from build123d import *

# Parameters (mm, degrees)
SKETCH1_R           = 42
SKETCH1_R_2         = 12
BOSS_EXTRUDE1_DEPTH = 10
CHAMFER1_SIZE       = 1.5


with BuildPart() as part:
    # Sketch1 → Boss-Extrude1 (new, symmetric)
    with BuildSketch(Plane(origin=(0, 0, 0), x_dir=(1, 0, 0), z_dir=(0, 1, 0))):
        with Locations(Location((0, 0, 0), (0, 0, 270))):
            Circle(SKETCH1_R)
        with Locations(Location((0, 0, 0), (0, 0, 270))):
            Circle(SKETCH1_R_2, mode=Mode.SUBTRACT)
    extrude(amount=BOSS_EXTRUDE1_DEPTH, both=True)

    # Sketch6 → Cut-Revolve11 (revolve, cut)
    with BuildSketch(Plane.XY, mode=Mode.PRIVATE) as cut_revolve11_sk:
        with BuildLine():
            Line((-42, 5.764577254), (-42, -5.764577254))
            ThreePointArc((-42, -5.764577254), (-36.235422746, 0), (-42, 5.764577254))
        make_face()
    revolve(cut_revolve11_sk.sketch.rotate(Axis((0, 0, 0), (0, 1, 0)), 180), axis=Axis((0, 0, 0), (0, 1, 0)), mode=Mode.SUBTRACT)

    # Chamfer1
    # the kernel refuses this chamfer: 1.5 mm, written as the material it takes off along each edge
    with BuildSketch(Plane(origin=(0, -5.764577254, 0), x_dir=(0, 0, 1), z_dir=(-1, 0, 0))) as chamfer1_piece_1:
        with BuildLine():
            Line((42, -CHAMFER1_SIZE), (40.217482923, 0.282517077))
            ThreePointArc((40.217482923, 0.282517077), (41.073277318, 0.074978324), (42, 0))
            Line((42, 0), (42, -CHAMFER1_SIZE))
        make_face()
    revolve(axis=Axis((0, -5.764577254, 0), (0, 1, 0)), revolution_arc=90, mode=Mode.SUBTRACT)
    with BuildSketch(Plane(origin=(0, 5.764577254, 0), x_dir=(1, 0, 0), z_dir=(0, 0, 1))) as chamfer1_piece_2:
        with BuildLine():
            Line((40.217482923, -0.282517077), (42, CHAMFER1_SIZE))
            Line((42, CHAMFER1_SIZE), (42, 0))
            ThreePointArc((42, 0), (41.073277318, -0.074978324), (40.217482923, -0.282517077))
        make_face()
    revolve(axis=Axis((0, 5.764577254, 0), (0, 1, 0)), revolution_arc=270, mode=Mode.SUBTRACT)
    with BuildSketch(Plane(origin=(0, -10, 0), x_dir=(0, 0, 1), z_dir=(-1, 0, 0))) as chamfer1_piece_3:
        Polygon((42, CHAMFER1_SIZE), (42 - CHAMFER1_SIZE, 0), (42, 0), align=None)
    revolve(axis=Axis((0, -10, 0), (0, 1, 0)), mode=Mode.SUBTRACT)
    with BuildSketch(Plane(origin=(0, 10, 0), x_dir=(0, 0, 1), z_dir=(-1, 0, 0))) as chamfer1_piece_4:
        Polygon((42, -CHAMFER1_SIZE), (42 - CHAMFER1_SIZE, 0), (42, 0), align=None)
    revolve(axis=Axis((0, 10, 0), (0, 1, 0)), mode=Mode.SUBTRACT)
    with BuildSketch(Plane(origin=(0, -10, 0), x_dir=(0, 0, 1), z_dir=(-1, 0, 0))) as chamfer1_piece_5:
        Polygon((12 + CHAMFER1_SIZE, 0), (12, CHAMFER1_SIZE), (12, 0), align=None)
    revolve(axis=Axis((0, -10, 0), (0, 1, 0)), mode=Mode.SUBTRACT)
    with BuildSketch(Plane(origin=(0, 10, 0), x_dir=(0, 0, 1), z_dir=(-1, 0, 0))) as chamfer1_piece_6:
        Polygon((12, -CHAMFER1_SIZE), (12 + CHAMFER1_SIZE, 0), (12, 0), align=None)
    revolve(axis=Axis((0, 10, 0), (0, 1, 0)), mode=Mode.SUBTRACT)
    with BuildSketch(Plane(origin=(0, 5.764577254, 0), x_dir=(0, 0, 1), z_dir=(-1, 0, 0))) as chamfer1_piece_7:
        with BuildLine():
            Line((40.217482923, -0.282517077), (42, CHAMFER1_SIZE))
            Line((42, CHAMFER1_SIZE), (42, 0))
            ThreePointArc((42, 0), (41.073277318, -0.074978324), (40.217482923, -0.282517077))
        make_face()
    revolve(axis=Axis((0, 5.764577254, 0), (0, 1, 0)), revolution_arc=90, mode=Mode.SUBTRACT)
    with BuildSketch(Plane(origin=(0, -5.764577254, 0), x_dir=(1, 0, 0), z_dir=(0, 0, 1))) as chamfer1_piece_8:
        with BuildLine():
            Line((42, -CHAMFER1_SIZE), (40.217482923, 0.282517077))
            ThreePointArc((40.217482923, 0.282517077), (41.073277318, 0.074978324), (42, 0))
            Line((42, 0), (42, -CHAMFER1_SIZE))
        make_face()
    revolve(axis=Axis((0, -5.764577254, 0), (0, 1, 0)), revolution_arc=270, mode=Mode.SUBTRACT)


solid = part.part
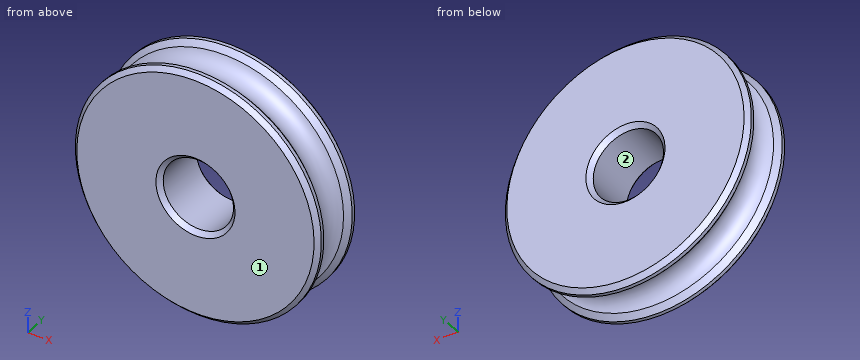
Can you work these out from the model? Positions are in its coordinate system, mm. Face numbers are marked on the shaded views. Coordinates: 2 decimals unless noted, no trailing zeros. Write each loop counter-clockwise with the first axis right and the second up, starting at its lowest first coordinate (ties: lowest second). Pieces come first, ordered by that corner, then holes. Notation, with made-up numbers: M 81.5,35.5 L 128.5,35.5 A30 ccw 128.5,72.5 Z; hole C 12,76.25 d4. An arc over 180 degrees is marked long. Use one line per item in the form item = value.
Q1. If we section it at B-B (x = 0): Write out the boundary of the cut face in (y, z).
Model answer:
outline = M -10,-40.5 L -8.5,-42 L -7.26,-42 L -5.48,-40.22 A5.76 cw 5.48,-40.22 L 7.26,-42 L 8.5,-42 L 10,-40.5 L 10,-13.5 L 8.5,-12 L -8.5,-12 L -10,-13.5 Z; M -10,13.5 L -8.5,12 L 8.5,12 L 10,13.5 L 10,40.5 L 8.5,42 L 7.26,42 L 5.48,40.22 A5.76 cw -5.48,40.22 L -7.26,42 L -8.5,42 L -10,40.5 Z
Q2. If we section it at C-C (y = -4.5): Write out the boundary of the cut face in (x, z), then the cut area to 3 significant figures.
Model answer:
outline = C 0,0 d76.79; hole C 0,0 d24
area = 4,180 mm^2
Q3. We'd pull the mould along Z, two halves only. Please class the marked faces 1 and 2: +Z half, -Z half, draft (parallel to the pull), parting line (faces both ways), or undercut.
Model answer:
face_1 = draft
face_2 = undercut
Q4. If we section it at A-A (z = 0): Write out the boundary of the cut face in (x, y).
Model answer:
outline = M -42,-8.5 L -40.5,-10 L -13.5,-10 L -12,-8.5 L -12,8.5 L -13.5,10 L -40.5,10 L -42,8.5 L -42,7.26 L -40.22,5.48 A5.76 cw -40.22,-5.48 L -42,-7.26 Z; M 12,-8.5 L 13.5,-10 L 40.5,-10 L 42,-8.5 L 42,-7.26 L 40.22,-5.48 A5.76 cw 40.22,5.48 L 42,7.26 L 42,8.5 L 40.5,10 L 13.5,10 L 12,8.5 Z
Q5. For P1, Ø4, axis at y = 0, z = 24.5, coming from the -X side; P2, Ø1.5, axis at y = -4, z = 1, coming from the -X side; P3, Ø1, axis at y = -7, z = 18.5, coming from the +X side, each with a flat end and sliding along its axis, tell me the tip position at first contact or that it passes through.
Model answer:
P1 = -28.4
P2 = -38.72
P3 = 37.91
Q6. I need wall thicknesses on line 1 along Z through (x, y) = (-6, 6); line 2 along Y through (x, z) = (28, 28.5); line 3 along Z through (x, y) = (-2.5, 1.5). Which ranges of each line are inside material? Lowest first, please. Write a range as from..to.
Model answer:
line_1 = -40.29..-10.39, 10.39..40.29
line_2 = -10..-5.39, 5.39..10
line_3 = -36.35..-11.74, 11.74..36.35
